```python
from build123d import *

# Parameters (mm, degrees)
SKETCH1_R           = 12.5
GEARBOX_DEPTH       = 22
SKETCH2_R           = 12.2
CAN_DEPTH           = 31
SKETCH3_R           = 11
END_CAP_DEPTH       = 3
SKETCH4_R           = 3.5
BEARING_BOSS_DEPTH  = 2
SHAFT_4MM_D_DEPTH   = 8
SKETCH6_R           = 1.25
M3_FACE_HOLES_DEPTH = 5


with BuildPart() as part:
    # Sketch1 → Gearbox (new body)
    with BuildSketch(Plane.XY.offset(-22)):
        Circle(SKETCH1_R)
    extrude(amount=GEARBOX_DEPTH)

    # Sketch2 → Can (add)
    with BuildSketch(Plane.XY.offset(-53)):
        Circle(SKETCH2_R)
    extrude(amount=CAN_DEPTH)

    # Sketch3 → End_cap (add)
    with BuildSketch(Plane.XY.offset(-56)):
        Circle(SKETCH3_R)
    extrude(amount=END_CAP_DEPTH)

    # Sketch4 → Bearing_boss (add)
    with BuildSketch(Plane.XY):
        Circle(SKETCH4_R)
    extrude(amount=BEARING_BOSS_DEPTH)

    # Sketch5 → Shaft_4mm_D (add)
    with BuildSketch(Plane.XY.offset(2)):
        with BuildLine():
            Line((1.45, -1.377497731), (1.45, 1.377497731))
            ThreePointArc((1.45, 1.377497731), (-2, 0), (1.45, -1.377497731))
        make_face()
    extrude(amount=SHAFT_4MM_D_DEPTH)

    # Sketch6 → M3_face_holes (cut)
    with BuildSketch(Plane.XY):
        with Locations((-8.5, 0)):
            Circle(SKETCH6_R)
        with Locations((8.5, 0)):
            Circle(SKETCH6_R)
    extrude(amount=-M3_FACE_HOLES_DEPTH, mode=Mode.SUBTRACT)


solid = part.part
```
Here's how the part is built. I have some questions about the finished solid (model axes, mm). A direction names the side the tool comes from. Give positions to 0.01 mm unless a question says otherwise; leave off trailing zeros. Write each loop counter-clockwise with the first axis right and the second up, starting at its lowest first coordinate (ties: lowest second). Pieces come first, ordered by that corner, then holes.
(1) Will these pins go through, and if not, where does the flat tip stop? pin 1 (1.5 mm diameter, centred on x = 2.5, y = 5.5, fed in from +Z); pin 2 (1.4 mm diameter, centred on y = -0.5, z = 6, fed in from +X); pin 3 (12.5 mm diameter, centred on x = 6, y = -2.5, fed in from +Z); pin 4 (1.2 mm diameter, centred on x = 8.5, y = 0, fed in from +Z).
Output values:
pin 1: stops at z = 0
pin 2: stops at x = 1.45
pin 3: stops at z = 10
pin 4: stops at z = -5
(2) Imagine slicing it at B-B, the plane x = 0. Write out the boundary of the cut face in (y, z).
Output values:
outline: (-12.5, -22) - (-12.2, -22) - (-12.2, -53) - (-11, -53) - (-11, -56) - (11, -56) - (11, -53) - (12.2, -53) - (12.2, -22) - (12.5, -22) - (12.5, 0) - (3.5, 0) - (3.5, 2) - (2, 2) - (2, 10) - (-2, 10) - (-2, 2) - (-3.5, 2) - (-3.5, 0) - (-12.5, 0) - close
(3) On a 3-axis mill with a long thin cutter (end or side, diameter ignored), from which of +Z, -Z, +X, -X, +Y, -Y can I reach the whole of each face in a straight line? I mean faces 1 (the face through (-2, 11, -53)), 2 (the face through (0, 0, -56)), 3 (the face through (-9, 0, -5)). Say none if no direction works.
Output values:
face 1: -Z
face 2: -Z, +X, -X, +Y, -Y
face 3: +Z
(4) Imagine slicing it at A-A, the plane y = 0. Write out the boundary of the cut face in (x, z).
Output values:
outline: (-12.5, -22) - (-12.2, -22) - (-12.2, -53) - (-11, -53) - (-11, -56) - (11, -56) - (11, -53) - (12.2, -53) - (12.2, -22) - (12.5, -22) - (12.5, 0) - (9.75, 0) - (9.75, -5) - (7.25, -5) - (7.25, 0) - (3.5, 0) - (3.5, 2) - (1.45, 2) - (1.45, 10) - (-2, 10) - (-2, 2) - (-3.5, 2) - (-3.5, 0) - (-7.25, 0) - (-7.25, -5) - (-9.75, -5) - (-9.75, 0) - (-12.5, 0) - close
(5) Imagine slicing it at C-C, the plane z = -9. Write out the boundary of the cut face in (x, y).
Output values:
outline: circle Ø25 at (0, 0)
(6) Imagine slicing it at D-D, the plane y = 7.25. Write out the boundary of the cut face in (x, z).
Output values:
outline: (-10.18, -22) - (-9.81, -22) - (-9.81, -53) - (-8.27, -53) - (-8.27, -56) - (8.27, -56) - (8.27, -53) - (9.81, -53) - (9.81, -22) - (10.18, -22) - (10.18, 0) - (-10.18, 0) - close
(7) If I drill on L1, parallel to Z at x = -9, y = 3.25; L2, parallel to X at y = -0.25, z = -15; L3, parallel to Z at x = -6.25, y = 10.25, over which ranges is the centre line in solid material (lowest first)?
Output values:
L1: z = -56 to 0
L2: x = -12.5 to 12.5
L3: z = -53 to 0
(8) Thinking about a two-plate mould opening in Y: for faces 4 (the face through (1.45, 0, 6)), 5 (the face through (3.233, -1.341, 0.986)), 6 (the face through (8, 0, -5)), which applies, pulls with the +Y half, pulls with the -Y half, needs draft (parallel to the pull), parting line crosses it, or undercut?
Output values:
face 4: needs draft
face 5: parting line crosses it
face 6: undercut
